Geometry check sheet. Reference: drawing and pictorial views, mm from the part's lowest x, y, z. A direction names the side the tool comes from. Give positions to 0.01 mm unless a question says otherwise; leave off trailing zeros. Write each loop counter-clockwise with the first axis right and the second up, starting at its lowest first coordinate (ties: lowest second). Pieces come first, ordered by that corner, then holes.
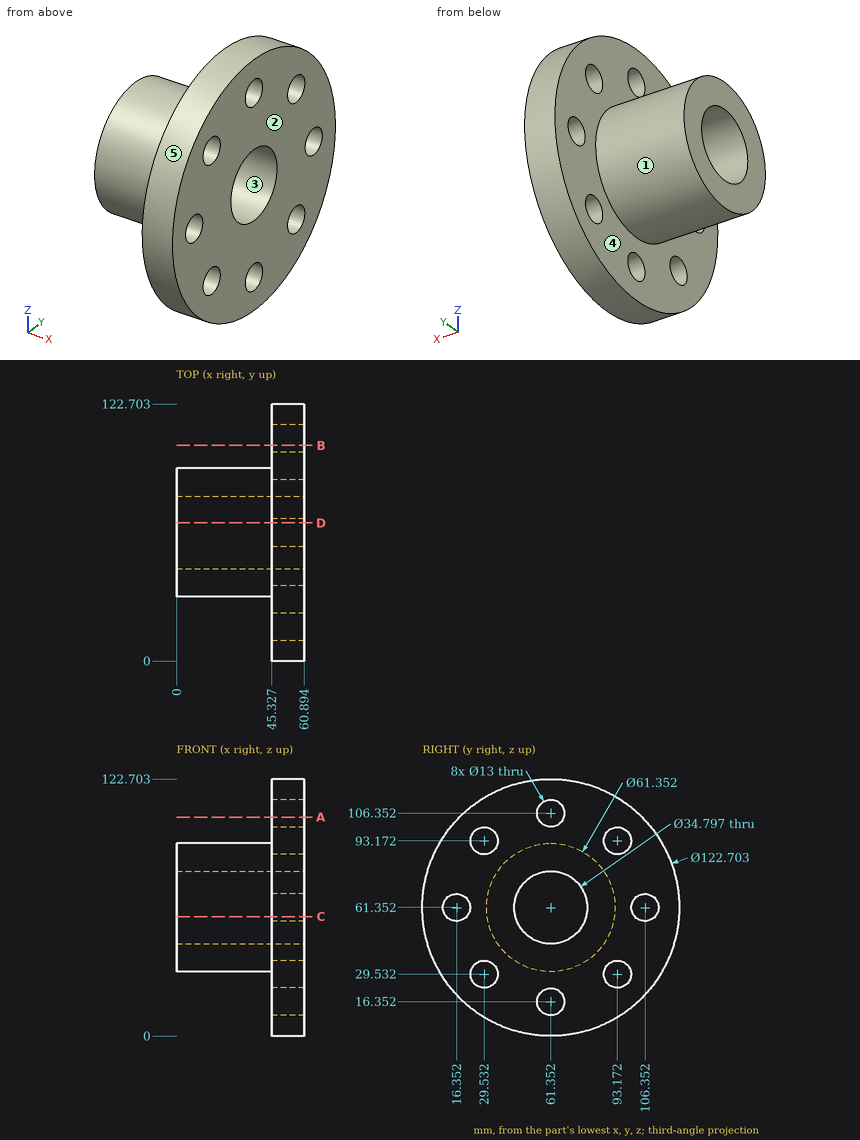
Item 1: Sectioned sample at C-C on z = 57. Record the cut outline in (x, y) (1 decimal).
Answer key:
outline: (0, 31) - (45.3, 31) - (45.3, 21.2) - (60.9, 21.2) - (60.9, 44.5) - (0, 44.5) - close; (0, 78.2) - (60.9, 78.2) - (60.9, 101.5) - (45.3, 101.5) - (45.3, 91.7) - (0, 91.7) - close; (45.3, 0.2) - (60.9, 0.2) - (60.9, 11.5) - (45.3, 11.5) - close; (45.3, 111.2) - (60.9, 111.2) - (60.9, 122.5) - (45.3, 122.5) - close
Item 2: Set-up check for the marked faces 4 and 5: record each of +Z, -Z, +X, -X, +Y, -Y from which the full face is reachable in a straight line by a thin tool's end or side.
Answer key:
face 4: -X
face 5: +X, -X
Item 3: Release check for a two-part mould opening along Y. For the marked faces 1, 2 and 3 record: released by +Y, released by -Y, zero draft, split by the parting line, or undercut.
Answer key:
face 1: split by the parting line
face 2: zero draft
face 3: undercut
Item 4: Sectioned sample at A-A on z = 104.5. Record the cut outline in (x, y), then the cut area to 3 significant figures.
Answer key:
outline: (45.33, 17.74) - (60.89, 17.74) - (60.89, 55.12) - (45.33, 55.12) - close; (45.33, 67.58) - (60.89, 67.58) - (60.89, 104.97) - (45.33, 104.97) - close
area: 1,160 mm2
Item 5: Depth check by flat-ended pin: pin 1 (8 mm diameter, centred on y = 29.53, z = 93.17, fed in from +X); pin 2 (3 mm diameter, centred on x = 34.5, z = 74, fed in from +Y); pin 3 (5 mm diameter, centred on x = 33, y = 34, fed in from -Z); pin 4 (2 mm diameter, centred on x = 38.5, z = 37.5, fed in from +Y) (1 decimal). Enter the tip coordinate at first touch or a pass-through.
Answer key:
pin 1: passes through
pin 2: stops at y = 89.93
pin 3: stops at z = 43.37
pin 4: stops at y = 81.8
Item 6: Sectioned sample at B-B on y = 103. Record the cut outline in (x, z).
Answer key:
outline: (45.33, 16.3) - (60.89, 16.3) - (60.89, 55.78) - (45.33, 55.78) - close; (45.33, 66.92) - (60.89, 66.92) - (60.89, 106.4) - (45.33, 106.4) - close
Item 7: Sectioned sample at D-D on y = 66. Record the cut outline in (x, z) (1 decimal).
Answer key:
outline: (0, 31) - (45.3, 31) - (45.3, 20.9) - (60.9, 20.9) - (60.9, 44.6) - (0, 44.6) - close; (0, 78.1) - (60.9, 78.1) - (60.9, 101.8) - (45.3, 101.8) - (45.3, 91.7) - (0, 91.7) - close; (45.3, 0.2) - (60.9, 0.2) - (60.9, 11.8) - (45.3, 11.8) - close; (45.3, 110.9) - (60.9, 110.9) - (60.9, 122.5) - (45.3, 122.5) - close
Item 8: Scan lines: line 1 along Z through (x, y) = (45, 51) (1 decimal); line 2 along Y through (x, z) = (47, 101) (1 decimal); line 3 along Y through (x, z) = (51, 97) (1 decimal). Record each from-to range of solid material in increasing order.
Answer key:
line 1: z = 32.5 to 47.4, 75.3 to 90.2
line 2: y = 14.5 to 57.7, 65 to 108.2
line 3: y = 11.4 to 24.3, 34.8 to 87.9, 98.4 to 111.3
